Read the model definition and answer for the solid it produces. Units are mm, in the model's axes. Face numbers are marked on the shaded views. A direction names the side the tool comes from. Coordinates: 2 decimals unless noted, no trailing zeros. Loops run counter-clockwise (first coordinate to the right, second up) from the corner with the lowest first, then second, coordinate; pieces in that order, holes last. Notation, with made-up numbers: M 47,46 L 68,46 A11 ccw 68,65 Z; hole C -8.75,-7.5 d2. An arc over 180 degrees is marked long. One line per item, written item: value. Start each with the question number.
1. The part is cut by section A-A (z = 27.5). Write down the section's boundary in (x, y), then the cut area to 3 significant figures.
2. The part is cut by section D-D (x = 18). Write down the section's boundary in (y, z).
3. Flat-ended cylindrical pins translate along their axes: pin 1 (6 mm diameter, centred on x = -30.5, z = 7.5, fed in from +Y); pin 2 (0.5 mm diameter, centred on y = 4.5, z = -27.5, fed in from +X); pin 3 (3 mm diameter, centred on y = 9, z = 4, fed in from -X). Find the tip coordinate at first contact, or state that the pin passes through.
4. The part is cut by section C-C (x = 46.5). Write down the section's boundary in (y, z).
5. The part is cut by section B-B (y = -1.25). State how many separate pieces and enclosed holes the cut face has, then the cut area to 3 significant figures.
6. Consider probe 1 along Z at (x, y) = (-46.5, 0.8); probe 2 along X at (y, z) = (10.5, -11); probe 3 along Z at (x, y) = (11, 10.25). Determine where each line is inside the solid, lowest interval first.
7. Determine the mould class of the marked faces 1, 2 and 3 for opening direction X: +X half, -X half, draft (parallel to the pull), parting line (faces both ways), or undercut.
8. For the marked faces 4, 5 and 6, determine the directions among +Z, -Z, +X, -X, +Y, -Y from which every point of the face is accessible in a straight line to the end or side of a thin tool.
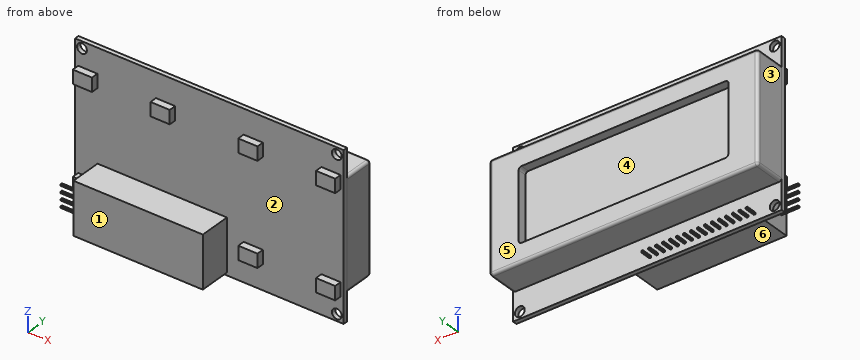
```python
from build123d import *

# Parameters (mm, degrees)
SKETCH1_W               = 98
SKETCH1_H               = 60
BOSS_EXTRUDE1_DEPTH     = 1.6
CUT_EXTRUDE1_START      = -2.6
SKETCH2_R               = 1.8
CUT_EXTRUDE1_DEPTH      = 3.6
SKETCH5_W               = 7
SKETCH5_H               = 5
BOSS_EXTRUDE3_DEPTH     = 2.57
MIRROR2_START           = -2.6
MIRROR2_COPY_1_SKETCH_R = 1.8
MIRROR2_COPY_1_DEPTH    = 3.6
MIRROR2_COPY_2_SKETCH_W = 7
MIRROR2_COPY_2_SKETCH_H = 5
MIRROR2_COPY_2_DEPTH    = 2.57
SKETCH3_W               = 97.98
SKETCH3_H               = 40
BOSS_EXTRUDE2_DEPTH     = 11.3
SKETCH4_W               = 76.5
SKETCH4_H               = 26.5
CUT_EXTRUDE2_DEPTH      = 3.3
FILLET1_R               = 1
SKETCH6_W               = 47.2
SKETCH6_H               = 19
BOSS_EXTRUDE4_DEPTH     = 11.5
SKETCH7_W               = 0.6
SKETCH7_H               = 0.6
BOSS_EXTRUDE5_DEPTH     = 6.5
SKETCH9_W               = 0.6
SKETCH9_H               = 0.6
BOSS_EXTRUDE7_DEPTH     = 3.9
LPATTERN1_COUNT         = 16
LPATTERN1_PITCH         = 2.54


with BuildPart() as part:
    # Sketch1 → Boss-Extrude1 (new body)
    with BuildSketch(Plane(origin=(0, 0, 0), x_dir=(1, 0, 0), z_dir=(0, 1, 0))):
        Rectangle(SKETCH1_W, SKETCH1_H)
    extrude(amount=BOSS_EXTRUDE1_DEPTH)

    # Sketch2 → Cut-Extrude1 (cut)
    with BuildSketch(Plane(origin=(0, 1.6, 0), x_dir=(1, 0, 0), z_dir=(0, 1, 0)).offset(CUT_EXTRUDE1_START)):
        with Locations((-46.5, 27.5)):
            Circle(SKETCH2_R)
    cut_extrude1 = extrude(amount=CUT_EXTRUDE1_DEPTH, mode=Mode.SUBTRACT)

    # Sketch5 → Boss-Extrude3 (add)
    with BuildSketch(Plane.XZ):
        with Locations((-44.375, 18.5)):
            Rectangle(SKETCH5_W, SKETCH5_H)
        with Locations((-16, 18.5)):
            Rectangle(SKETCH5_W, SKETCH5_H)
    boss_extrude3 = extrude(amount=BOSS_EXTRUDE3_DEPTH)

    # Mirror1: Cut-Extrude1, Boss-Extrude3 across plane
    add(cut_extrude1.mirror(Plane.XY), mode=Mode.SUBTRACT)
    add(boss_extrude3.mirror(Plane.XY))

    # Mirror2: Cut-Extrude1, Boss-Extrude3 across plane
    add(cut_extrude1.mirror(Plane(origin=(0, 0, 0), x_dir=(0, 0, 1), z_dir=(1, 0, 0))), mode=Mode.SUBTRACT)
    add(boss_extrude3.mirror(Plane(origin=(0, 0, 0), x_dir=(0, 0, 1), z_dir=(1, 0, 0))))

    # Mirror2 copy 1 sketch → Mirror2 copy 1 (cut)
    with BuildSketch(Plane(origin=(0, 1.6, 0), x_dir=(-1, 0, 0), z_dir=(0, 1, 0)).offset(MIRROR2_START)):
        with Locations((-46.5, 27.5)):
            Circle(MIRROR2_COPY_1_SKETCH_R)
    extrude(amount=MIRROR2_COPY_1_DEPTH, mode=Mode.SUBTRACT)

    # Mirror2 copy 2 sketch → Mirror2 copy 2 (add)
    with BuildSketch(Plane(origin=(0, 0, 0), x_dir=(-1, 0, 0), z_dir=(0, -1, 0))):
        with Locations((-44.375, 18.5)):
            Rectangle(MIRROR2_COPY_2_SKETCH_W, MIRROR2_COPY_2_SKETCH_H)
        with Locations((-16, 18.5)):
            Rectangle(MIRROR2_COPY_2_SKETCH_W, MIRROR2_COPY_2_SKETCH_H)
    extrude(amount=MIRROR2_COPY_2_DEPTH)

    # Sketch3 → Boss-Extrude2 (add)
    with BuildSketch(Plane(origin=(0, 1.6, 0), x_dir=(1, 0, 0), z_dir=(0, 1, 0))):
        Rectangle(SKETCH3_W, SKETCH3_H)
    extrude(amount=BOSS_EXTRUDE2_DEPTH)

    # Sketch4 → Cut-Extrude2 (cut)
    with BuildSketch(Plane(origin=(0, 12.9, 0), x_dir=(1, 0, 0), z_dir=(0, 1, 0))):
        Rectangle(SKETCH4_W, SKETCH4_H)
    extrude(amount=-CUT_EXTRUDE2_DEPTH, mode=Mode.SUBTRACT)

    # Fillet1
    fillet1_edges = [part.edges().sort_by_distance(p)[0] for p in [
        (48.99, 7.25, 20),
        (48.99, 7.25, -20),
        (-48.99, 7.25, -20),
        (-48.99, 7.25, 20),
        (48.99, 12.9, 0),
        (0, 12.9, -20),
        (-48.99, 12.9, 0),
        (0, 12.9, 20),
        (38.25, 11.25, -13.25),
        (38.25, 11.25, 13.25),
        (-38.25, 11.25, 13.25),
        (-38.25, 11.25, -13.25),
    ]]
    fillet(fillet1_edges, radius=FILLET1_R)

    # Sketch6 → Boss-Extrude4 (add)
    with BuildSketch(Plane.XZ):
        with Locations((-17.2, -19.5)):
            Rectangle(SKETCH6_W, SKETCH6_H)
    extrude(amount=BOSS_EXTRUDE4_DEPTH)

    # Sketch7 → Boss-Extrude5 (add)
    with BuildSketch(Plane(origin=(-40.8, 0, 0), x_dir=(0, 0, -1), z_dir=(1, 0, 0))):
        with Locations((15.25, -8.8)):
            Rectangle(SKETCH7_W, SKETCH7_H)
        with Locations((17.79, -8.8)):
            Rectangle(SKETCH7_W, SKETCH7_H)
        with Locations((20.33, -8.8)):
            Rectangle(SKETCH7_W, SKETCH7_H)
        with Locations((22.87, -8.8)):
            Rectangle(SKETCH7_W, SKETCH7_H)
    extrude(amount=-BOSS_EXTRUDE5_DEPTH)

    # Sketch9 → Boss-Extrude7 (add)
    with BuildSketch(Plane(origin=(0, 1.6, 0), x_dir=(1, 0, 0), z_dir=(0, 1, 0))):
        with Locations((-39.2, 27.46)):
            Rectangle(SKETCH9_W, SKETCH9_H)
    boss_extrude7 = extrude(amount=BOSS_EXTRUDE7_DEPTH)

    # LPattern1: Boss-Extrude7 ×16
    with Locations(*[(i * LPATTERN1_PITCH, 0, 0) for i in range(1, LPATTERN1_COUNT)]):
        add(boss_extrude7)


solid = part.part
```
Answer block:
1. outline: M -49,0 L -48.3,0 L -48.3,1.6 L -49,1.6 Z; M -44.7,0 L 44.7,0 L 44.7,1.6 L -44.7,1.6 Z; M 48.3,0 L 49,0 L 49,1.6 L 48.3,1.6 Z
1. area: 145 mm2
2. outline: M -2.57,-21 L 0,-21 L 0,-30 L 1.6,-30 L 1.6,-20 L 11.9,-20 A1 ccw 12.9,-19 L 12.9,-13.25 L 9.6,-13.25 L 9.6,13.25 L 12.9,13.25 L 12.9,19 A1 ccw 11.9,20 L 1.6,20 L 1.6,30 L 0,30 L 0,21 L -2.57,21 L -2.57,16 L 0,16 L 0,-16 L -2.57,-16 Z
3. pin 1: stops at y = 9.6
3. pin 2: stops at x = -0.8
3. pin 3: stops at x = -48.99
4. outline: M -2.57,-21 L 0,-21 L 0,-25.7 L 1.6,-25.7 L 1.6,-20 L 11.9,-20 A1 ccw 12.9,-19 L 12.9,19 A1 ccw 11.9,20 L 1.6,20 L 1.6,25.7 L 0,25.7 L 0,21 L -2.57,21 L -2.57,16 L 0,16 L 0,-16 L -2.57,-16 Z; M 0,-30 L 1.6,-30 L 1.6,-29.3 L 0,-29.3 Z; M 0,29.3 L 1.6,29.3 L 1.6,30 L 0,30 Z
5. separate pieces: 8
5. enclosed holes: 0
5. area: 1,140 mm2
6. probe 1: z = -30 to -29.3, -25.7 to 25.7, 29.3 to 30
6. probe 2: x = -48.99 to -38.25, 38.25 to 48.99
6. probe 3: z = -20 to -13.25, 13.25 to 20
7. face 1: draft
7. face 2: undercut
7. face 3: -X half
8. face 4: +Y
8. face 5: +Z, -Z, +X, -X, +Y
8. face 6: -Z, +X, -X, -Y
